```python
from build123d import *

# Parameters (mm, degrees)
F1_DEPTH = 19.05
F2_R     = 2.54
F3_DEPTH = 9.525
F4_DEPTH = 9.525


with BuildPart() as f1:
    # F0 (on Front) → F1 (new body)
    with BuildSketch(Plane.XZ):
        Polygon((-38.1, 65.991136), (-76.2, 0), (0, 0), align=None)
    extrude(amount=F1_DEPTH)

    # F2 (on face) → F3 (cut)
    with BuildSketch(Plane.XZ.offset(19.05)):
        with Locations((-62.770836, 6.895666)):
            Circle(F2_R)
    extrude(amount=-F3_DEPTH, mode=Mode.SUBTRACT)

    # F2 (on face) → F4 (cut)
    with BuildSketch(Plane.XZ.offset(19.05)):
        with Locations((-38.1, 6.895666)):
            Circle(F2_R)
        with Locations((-62.770836, 6.895666)):
            Circle(F2_R)
        with Locations((-49.385134, 6.895666)):
            Circle(F2_R)
        with Locations((-25.858745, 6.895666)):
            Circle(F2_R)
        with Locations((-13.284297, 6.895666)):
            Circle(F2_R)
        with Locations((-56.686427, 19.470114)):
            Circle(F2_R)
        with Locations((-44.111978, 19.470114)):
            Circle(F2_R)
        with Locations((-31.131901, 19.470114)):
            Circle(F2_R)
        with Locations((-20.788403, 19.470114)):
            Circle(F2_R)
        with Locations((-38.1, 33.667073)):
            Circle(F2_R)
        with Locations((-49.385134, 33.667073)):
            Circle(F2_R)
        with Locations((-27.684068, 33.667073)):
            Circle(F2_R)
        with Locations((-44.111978, 45.633078)):
            Circle(F2_R)
        with Locations((-38.1, 54.354072)):
            Circle(F2_R)
        with Locations((-32.957226, 45.633078)):
            Circle(F2_R)
    extrude(amount=-F4_DEPTH, mode=Mode.SUBTRACT)


solid = f1.part
```
Geometry: final body of the model. Coordinates: model frame, mm. A direction names the side the tool comes from. Round coordinates to 2 decimals unless told otherwise and drop trailing zeros. Loops run counter-clockwise (first coordinate to the right, second up) from the corner with the lowest first, then second, coordinate; pieces in that order, holes last. Notation, with made-up numbers: (-21, 34.5) -> (1, 34.5) arc R25 ccw to (1, 49.5) -> close; hole circle Ø11 at (-21, 15.5). An arc over 180 degrees is marked (long way). Use one line per item in the form item = value. Start each with the question number.
1) Access query for faces 4 (the flat face through (-39, 0, 26)), 5 (the flat face through (-28, -9.525, 34)). Directions: +Z, -Z, +X, -X, +Y, -Y. A direction counts if a zero-diameter tool reaches every point of the face in a straight line with its end or side. Return the directions, or none.
2) Line query: L1, parallel to Z at x = -27.5, y = -10; L2, parallel to X at y = -18, z = 20; L3, parallel to Z at x = -25, y = -13. Output: solid intervals per line, ascending.
3) Section A-A on z = 8.5. Output: boundary loops of the cut face in (x, y) (3 decimals).
4) Draft query along Z for faces 1 (the cylindrical face through (-38.7, -14.4, 31.2)), 2 (the flat face through (-18.78, -9.39, 32.53)), 3 (the flat face through (-39, -19.05, 19)). Return one class per face: released by +Z, released by -Z, zero draft, split by the parting line, or undercut.
5) First-contact query: P1, Ø1, axis at y = -3.5, z = 32, coming from the -X side; P2, Ø3, axis at x = -31.13, z = 19.47, coming from the -Y side (3 decimals); P3, Ø4, axis at y = -12.5, z = 53, coming from the -X side; P4, Ø8, axis at x = -52, z = 54, coming from the +Y side. Flat tips, straight axial feed; report the tip coordinate or a pass-through.
6) Section C-C on y = -6. Output: boundary loops of the cut face in (x, z).
7) Section D-D on z = 47. Output: boundary loops of the cut face in (x, y) (3 decimals).
8) Section B-B on y = -13.5. Give the number of separate pieces and of enclosed holes in the cut face, then the cut area to 3 significant figures.
Response:
q1.face_4 = +Z, -Z, +X, -X, +Y
q1.face_5 = -Y
q2.L1 = 0 to 4.96, 8.83 to 31.13, 36.2 to 47.63
q2.L2 = -64.65 to -59.17, -54.2 to -46.6, -41.63 to -33.62, -28.65 to -23.27, -18.3 to -11.55
q2.L3 = 0 to 4.51, 9.29 to 43.3
q3.outline = (-71.293, -19.05) -> (-64.74, -19.05) -> (-64.74, -9.525) -> (-60.802, -9.525) -> (-60.802, -19.05) -> (-51.354, -19.05) -> (-51.354, -9.525) -> (-47.416, -9.525) -> (-47.416, -19.05) -> (-40.069, -19.05) -> (-40.069, -9.525) -> (-36.131, -9.525) -> (-36.131, -19.05) -> (-27.828, -19.05) -> (-27.828, -9.525) -> (-23.89, -9.525) -> (-23.89, -19.05) -> (-15.253, -19.05) -> (-15.253, -9.525) -> (-11.315, -9.525) -> (-11.315, -19.05) -> (-4.907, -19.05) -> (-4.907, 0) -> (-71.293, 0) -> close
q4.face_1 = undercut
q4.face_2 = released by +Z
q4.face_3 = zero draft
q5.P1 = -58.01
q5.P2 = -9.525
q5.P3 = -46.76
q5.P4 = through
q6.outline = (-76.2, 0) -> (0, 0) -> (-38.1, 65.99) -> close
q7.outline = (-49.065, -19.05) -> (-46.253, -19.05) -> (-46.253, -9.525) -> (-41.971, -9.525) -> (-41.971, -19.05) -> (-35.098, -19.05) -> (-35.098, -9.525) -> (-30.816, -9.525) -> (-30.816, -19.05) -> (-27.135, -19.05) -> (-27.135, 0) -> (-49.065, 0) -> close
q8.separate_pieces = 1
q8.enclosed_holes = 15
q8.area = 2,210 mm^2
